Can you work these out from the model? Positions are in its coordinate system, mm. A direction names the side the tool comes from. Coordinates: 2 decimals unless noted, no trailing zeros. Write each loop counter-clockwise with the first axis right and the second up, starting at its lowest first coordinate (ties: lowest second). Pieces come first, ordered by that corner, then holes. Notation, with made-up numbers: M 49,-7 L 92,-7 A15 ccw 92,2 Z; hole C -20.75,-7.75 d5. An arc over 180 degrees is marked long. Use one line per item in the form item = value. Start each with the question number.
```python
from build123d import *

# Parameters (mm, degrees)
SKETCH1_R           = 14
SKETCH1_W           = 6.85
SKETCH1_H           = 1.8
BOSS_EXTRUDE4_DEPTH = 1


with BuildPart() as part:
    # Sketch1 → Boss-Extrude4 (new body)
    with BuildSketch(Plane.XY):
        Circle(SKETCH1_R)
        with Locations((0.084285819, -9.827892173)):
            Rectangle(SKETCH1_W, SKETCH1_H, mode=Mode.SUBTRACT)
    extrude(amount=BOSS_EXTRUDE4_DEPTH)


solid = part.part
```
1) Suppose I cut it at A-A on x = 0. Please give me the cut outline in (y, z), and give its area (3 significant figures).
2) Suppose I cut it at D-D on y = -11.5. Please give me the cut outline in (x, z).
3) Suppose I cut it at B-B on z = 0.85. Please give me the cut outline in (x, y).
4) If we mould it in two halves opening along Y, with no side actions, what happens to faces 3 (the face through (0, 0, 0)), 4 (the face through (12.932, -5.362, 0.493)), 5 (the face through (0, -10.728, 0.5))? For each: +Y half, -Y half, draft (parallel to the pull), parting line (faces both ways), or undercut.
5) Suppose I cut it at C-C on x = 5. Please give me the cut outline in (y, z), and give its area (3 significant figures).
6) Please list where these lines run through material, in increasing order: line 1 (Y direction, x = -2, z = 0.5); line 2 (X direction, y = -9.75, z = 0.2); line 3 (Y direction, x = -6.25, z = 0.45).
7) Which directions (+Z, -Z, +X, -X, +Y, -Y) give clear straight access to the entire face, cutting with the end or side of a thin tool? Please do faces 1 (the face through (0, 0, 1)), 2 (the face through (0, -8.928, 0.5)).
Computed values:
q1.outline = M -14,0 L -10.73,0 L -10.73,1 L -14,1 Z; M -8.93,0 L 14,0 L 14,1 L -8.93,1 Z
q1.area = 26.2 mm²
q2.outline = M -7.98,0 L 7.98,0 L 7.98,1 L -7.98,1 Z
q3.outline = C 0,0 d28; hole M -3.34,-10.73 L 3.51,-10.73 L 3.51,-8.93 L -3.34,-8.93 Z
q4.face_3 = draft
q4.face_4 = parting line
q4.face_5 = undercut
q5.outline = M -13.08,0 L 13.08,0 L 13.08,1 L -13.08,1 Z
q5.area = 26.2 mm²
q6.line_1 = -13.86 to -10.73, -8.93 to 13.86
q6.line_2 = -10.05 to -3.34, 3.51 to 10.05
q6.line_3 = -12.53 to 12.53
q7.face_1 = +Z, +X, -X, +Y, -Y
q7.face_2 = +Z, -Z
